Geometry: final body of the model. Coordinates: model frame, mm. Give positions to 0.01 mm unless a question says otherwise; leave off trailing zeros. Order: outer loops, then holes, each group sorted by start corner. A loop starts at its lowest first (then second) coordinate and runs counter-clockwise, first axis right, second up. Notation, with made-up numbers: (8, 30.5) - (48, 30.5) arc R17 cw to (48, 51.5) - close; hole circle Ø2 at (73, -13.75). An arc over 180 degrees is marked (long way). One line per item, written item: value.
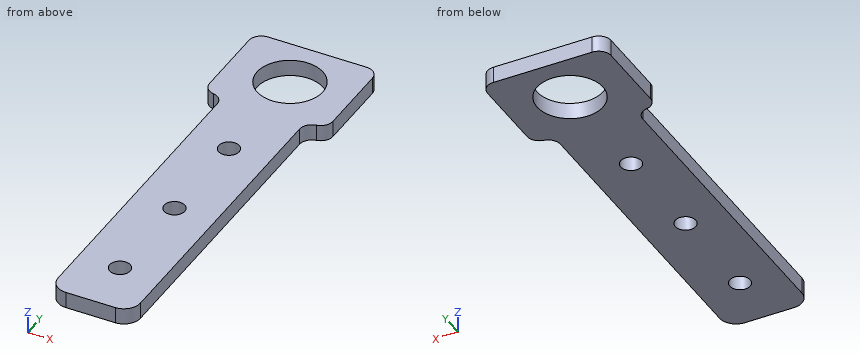
```python
from build123d import *

# Parameters (mm, degrees)
SKETCH_1_W          = 20
SKETCH_1_H          = 30
SKETCH_1_R          = 1.5
EXTRUDE_1_DEPTH     = 4
SKETCH_2_W          = 30
SKETCH_2_H          = 4
EXTRUDE_2_DEPTH     = 24
FILLET_1_R          = 3
SKETCH_3_R          = 8
CUT_EXTRUDE_1_DEPTH = 24
FILLET_2_R          = 3
SKETCH_4_R          = 1.5
EXTRUDE_3_DEPTH     = 4
SKETCH_9_R          = 2.5
CUT_EXTRUDE_2_DEPTH = 5.0000001
SKETCH_11_W         = 20
SKETCH_11_H         = 50
EXTRUDE_5_DEPTH     = 4
SKETCH_13_R         = 2.5
CUT_EXTRUDE_3_DEPTH = 10
FILLET_4_R          = 4
FILLET_5_R          = 4


with BuildPart() as part:
    # 草图1 → 凸台-拉伸1 (new body)
    with BuildSketch(Plane.XY):
        Rectangle(SKETCH_1_W, SKETCH_1_H)
        with Locations((-5, 3)):
            Circle(SKETCH_1_R, mode=Mode.SUBTRACT)
        with Locations((5, 3)):
            Circle(SKETCH_1_R, mode=Mode.SUBTRACT)
        with Locations((-5, -7)):
            Circle(SKETCH_1_R, mode=Mode.SUBTRACT)
        with Locations((5, -7)):
            Circle(SKETCH_1_R, mode=Mode.SUBTRACT)
    extrude(amount=EXTRUDE_1_DEPTH)

    # 草图2 → 凸台-拉伸2 (add)
    with BuildSketch(Plane(origin=(0, 15, 0), x_dir=(1, 0, 0), z_dir=(0, 1, 0))):
        with Locations((0, -2)):
            Rectangle(SKETCH_2_W, SKETCH_2_H)
    extrude(amount=EXTRUDE_2_DEPTH)

    # 圆角1
    fillet_1_edges = [part.edges().sort_by_distance(p)[0] for p in [
        (-10, 15, 2),
        (10, 15, 2),
    ]]
    fillet(fillet_1_edges, radius=FILLET_1_R)

    # 草图3 → 切除-拉伸1 (cut)
    with BuildSketch(Plane.XY.offset(4)):
        with Locations((0, 26.5)):
            Circle(SKETCH_3_R)
    extrude(amount=-CUT_EXTRUDE_1_DEPTH, mode=Mode.SUBTRACT)

    # 圆角2
    fillet_2_edges = [part.edges().sort_by_distance(p)[0] for p in [
        (15, 15, 2),
        (15, 39, 2),
        (-15, 39, 2),
        (-15, 15, 2),
    ]]
    fillet(fillet_2_edges, radius=FILLET_2_R)

    # 草图4 → 凸台-拉伸3 (add)
    with BuildSketch(Plane.XY.offset(4)):
        with Locations((5, 3)):
            Circle(SKETCH_4_R)
        with Locations((5, -7)):
            Circle(SKETCH_4_R)
        with Locations((-5, 3)):
            Circle(SKETCH_4_R)
        with Locations((-5, -7)):
            Circle(SKETCH_4_R)
    extrude(amount=-EXTRUDE_3_DEPTH)

    # 草图9 → 切除-拉伸2 (cut, through all)
    with BuildSketch(Plane.XY.offset(4)):
        with Locations((0, -1.5)):
            Circle(SKETCH_9_R)
    extrude(amount=-CUT_EXTRUDE_2_DEPTH, mode=Mode.SUBTRACT)

    # 草图11 → 凸台-拉伸5 (add)
    with BuildSketch(Plane.XY.offset(4)):
        with Locations((0, -40)):
            Rectangle(SKETCH_11_W, SKETCH_11_H)
    extrude(amount=-EXTRUDE_5_DEPTH)

    # 草图13 → 切除-拉伸3 (cut)
    with BuildSketch(Plane.XY.offset(4)):
        with Locations((0, -26.5)):
            Circle(SKETCH_13_R)
        with Locations((0, -51.5)):
            Circle(SKETCH_13_R)
    extrude(amount=-CUT_EXTRUDE_3_DEPTH, mode=Mode.SUBTRACT)

    # 圆角4
    fillet_4_edges = [part.edges().sort_by_distance(p)[0] for p in [
        (10, -65, 2),
    ]]
    fillet(fillet_4_edges, radius=FILLET_4_R)

    # 圆角5
    fillet_5_edges = [part.edges().sort_by_distance(p)[0] for p in [
        (-10, -65, 2),
    ]]
    fillet(fillet_5_edges, radius=FILLET_5_R)


solid = part.part
```
1) Section A-A, the plane x = 0. Return loops of the section in (y, z).
Answers below:
outline: (-65, 0) - (-54, 0) - (-54, 4) - (-65, 4) - close; (-49, 0) - (-29, 0) - (-29, 4) - (-49, 4) - close; (-24, 0) - (-4, 0) - (-4, 4) - (-24, 4) - close; (1, 0) - (18.5, 0) - (18.5, 4) - (1, 4) - close; (34.5, 0) - (39, 0) - (39, 4) - (34.5, 4) - close
2) Material intervals for line 1 along Y through (x, z) = (0, 1.8); line 2 along X through (y, z) = (-21.5, 2.9); line 3 along Y through (x, z) = (1, 3.5), sorted ascending.
Answers below:
line 1: -65 to -54, -49 to -29, -24 to -4, 1 to 18.5, 34.5 to 39
line 2: -10 to 10
line 3: -65 to -53.79, -49.21 to -28.79, -24.21 to -3.79, 0.79 to 18.56, 34.44 to 39
3) First-contact query: pin 1 (3 mm diameter, centred on x = -2.5, y = 20, fed in from +Z). Flat tip, straight axial feed; report the tip coordinate or a pass-through.
Answers below:
pin 1: z = 4
4) Section C-C, the plane x = 4.5. Return loops of the section in (y, z).
Answers below:
outline: (-65, 0) - (19.89, 0) - (19.89, 4) - (-65, 4) - close; (33.11, 0) - (39, 0) - (39, 4) - (33.11, 4) - close
5) Section B-B, the plane y = -26.5. Return loops of the section in (x, z), then the cut area to 3 significant figures.
Answers below:
outline: (-10, 0) - (-2.5, 0) - (-2.5, 4) - (-10, 4) - close; (2.5, 0) - (10, 0) - (10, 4) - (2.5, 4) - close
area: 60.0 mm^2
6) Section D-D, the plane z = 2. Count the separate pieces of the cut face and the enclosed holes in it, then the cut area to 3 significant figures.
Answers below:
separate pieces: 1
enclosed holes: 4
area: 2,050 mm^2
